from build123d import *

# Parameters (mm, degrees)
F0_W     = 101.6
F0_H     = 63.5
F1_DEPTH = 50.8
F2_R     = 6.35
F3_DEPTH = 50.801
F4_W     = 12.7
F4_H     = 38.1
F6_W     = 12.7
F6_H     = 5.855737


with BuildPart() as f1:
    # F0 (on Front) → F1 (new body)
    with BuildSketch(Plane.XZ):
        Rectangle(F0_W, F0_H)
    extrude(amount=-F1_DEPTH)

    # F2 (on face) → F3 (cut, through all)
    with BuildSketch(Plane.XZ):
        with Locations((38.1, -19.05)):
            Circle(F2_R)
        with Locations((38.1, 19.05)):
            Circle(F2_R)
        with Locations((-38.1, 19.05)):
            Circle(F2_R)
        with Locations((-38.1, -19.05)):
            Circle(F2_R)
    extrude(amount=-F3_DEPTH, mode=Mode.SUBTRACT)

    # F4 (on Top) → F5 (revolve)
    with BuildSketch(Plane.XY):
        with Locations((6.35, 69.85)):
            Rectangle(F4_W, F4_H)
    revolve(axis=Axis((0, 69.85, 0), (0, 1, 0)))

    # F6 (on Top) → F7 (revolve, cut)
    with BuildSketch(Plane.XY):
        with Locations((-14.233844, 60.077868)):
            Rectangle(F6_W, F6_H)
    revolve(axis=Axis((0, 88.9, 0), (0, 1, 0)), mode=Mode.SUBTRACT)


solid = f1.part
Check sheet for the modelled part. Datum: model origin and axes. Units: mm. A direction names the side the tool comes from. Coordinates: 2 decimals unless noted, no trailing zeros. Write each loop counter-clockwise with the first axis right and the second up, starting at its lowest first coordinate (ties: lowest second). Pieces come first, ordered by that corner, then holes.
Item 1: Access from +Z, -Z, +X, -X, +Y, -Y to the whole of each face (thin tool, end or side, straight path). Record for faces 5 (the face through (0.2, 63.006, -8.3)), 6 (the face through (31.756, 25.044, 19.329)), 7 (the face through (-2.75, 76.13, 12.4)).
Numbers:
face 5: none
face 6: +Y, -Y
face 7: +Y
Item 2: Cross-section at C-C on y = 18. Record the boundary of the cut face in (x, z), then the cut area to 3 significant figures.
Numbers:
outline: (-50.8, -31.75) - (50.8, -31.75) - (50.8, 31.75) - (-50.8, 31.75) - close; hole circle Ø12.7 at (-38.1, -19.05); hole circle Ø12.7 at (-38.1, 19.05); hole circle Ø12.7 at (38.1, -19.05); hole circle Ø12.7 at (38.1, 19.05)
area: 5,940 mm2
Item 3: Scan lines: probe 1 along X at (y, z) = (49, -19); probe 2 along Z at (x, y) = (-38.1, 15); probe 3 along X at (y, z) = (18.5, -14). Record each from-to range of solid material in increasing order.
Numbers:
probe 1: x = -50.8 to -44.45, -31.75 to 31.75, 44.45 to 50.8
probe 2: z = -31.75 to -25.4, -12.7 to 12.7, 25.4 to 31.75
probe 3: x = -50.8 to -41.95, -34.25 to 34.25, 41.95 to 50.8
Item 4: Cross-section at B-B on z = 19.05. Record the boundary of the cut face in (x, y).
Numbers:
outline: (-50.8, 0) - (-44.45, 0) - (-44.45, 50.8) - (-50.8, 50.8) - close; (-31.75, 0) - (31.75, 0) - (31.75, 50.8) - (-31.75, 50.8) - close; (44.45, 0) - (50.8, 0) - (50.8, 50.8) - (44.45, 50.8) - close
Item 5: Cross-section at D-D on x = 11. Record the boundary of the cut face in (y, z).
Numbers:
outline: (0, -31.75) - (50.8, -31.75) - (50.8, -6.35) - (57.15, -6.35) - (57.15, 6.35) - (50.8, 6.35) - (50.8, 31.75) - (0, 31.75) - close; (63.01, -6.35) - (88.9, -6.35) - (88.9, 6.35) - (63.01, 6.35) - close
Item 6: Cross-section at A-A on x = 38.1. Record the boundary of the cut face in (y, z).
Numbers:
outline: (0, -31.75) - (50.8, -31.75) - (50.8, -25.4) - (0, -25.4) - close; (0, -12.7) - (50.8, -12.7) - (50.8, 12.7) - (0, 12.7) - close; (0, 25.4) - (50.8, 25.4) - (50.8, 31.75) - (0, 31.75) - close
Item 7: Mould release check, pull along X, two halves, no side actions. Record for faces 1 (the face through (-1, 25, 31.75)), 2 (the face through (-32.043, 25.044, 20.957)), 3 (the face through (-32.234, 25.044, -21.482)), 4 (the face through (1.7, 60.1, -7.7)): released by +X, released by -X, zero draft, split by the parting line, or undercut.
Numbers:
face 1: zero draft
face 2: undercut
face 3: undercut
face 4: split by the parting line
Item 8: Depth check by flat-ended pin: pin 1 Ø20.5 at (x, z) = (38.1, 19.05) entering from +Y; pin 2 Ø6 at (y, z) = (64.5, -6) entering from +X; pin 3 Ø8 at (y, z) = (55.5, -11.5) entering from +X. Enter the tip coordinate at first touch or a pass-through.
Numbers:
pin 1: stops at y = 50.8
pin 2: stops at x = 12.34
pin 3: stops at x = 10.25
